Geometry check sheet. Reference: the model listing, model coordinates, mm. A direction names the side the tool comes from. Round coordinates to 2 decimals unless told otherwise and drop trailing zeros. Order: outer loops, then holes, each group sorted by start corner. A loop starts at its lowest first (then second) coordinate and runs counter-clockwise, first axis right, second up. Notation, with made-up numbers: M 5,29 L 41,29 A26 cw 41,45 Z; hole C 61,-9 d4. An arc over 180 degrees is marked long. Return JSON: item names as keys, results as strings. Group by question number.
```python
from build123d import *

# Parameters (mm, degrees)
F0_R            = 10
F0_R_2          = 8
F1_DEPTH        = 4
F3_DEPTH        = 3
F3_COPIES_COUNT = 3
F5_DEPTH        = 3
F5_COPIES_COUNT = 3
F7_DEPTH        = 3
F7_COPIES_COUNT = 3
F9_DEPTH        = 3
F9_COPIES_COUNT = 3
F10_W           = 0.5
F10_H           = 2
F10_W_2         = 3
F10_H_2         = 6


# Not quite as in the source:
# - a pattern or mirror of a feature is missing from the dataset's text; its kind, count and spacing are read off the source's solid


with BuildPart() as f1:
    # F0 (on Front) → F1 (new body, symmetric)
    with BuildSketch(Plane.XZ):
        Circle(F0_R)
        Circle(F0_R_2, mode=Mode.SUBTRACT)
    extrude(amount=F1_DEPTH, both=True)

    # F2 (on face) → F3 (cut)
    with BuildSketch(Plane.XZ.offset(4)):
        with BuildLine():
            Line((-0.525, 8.9827548503), (-0.525, 7.9827548503))
            ThreePointArc((-0.525, 7.9827548503), (0, 8), (0.525, 7.9827548503))
            Line((0.525, 7.9827548503), (0.525, 8.9827548503))
            Line((0.525, 8.9827548503), (-0.525, 8.9827548503))
        make_face()
    f3 = extrude(amount=-F3_DEPTH, mode=Mode.SUBTRACT)

    # F3_copies: F3 ×3 about axis
    f3_copies_axis = Axis((0, 0, 0), (0, 1, 0))
    for i in range(1, F3_COPIES_COUNT):
        add(f3.rotate(f3_copies_axis, i * 360 / F3_COPIES_COUNT), mode=Mode.SUBTRACT)

    # F4 (on Front) → F5 (cut)
    with BuildSketch(Plane.XZ):
        with BuildLine():
            ThreePointArc((6.6507684925, 4.4460407621), (6.9282032303, 4), (7.1757684925, 3.5367140882))
            Line((7.1757684925, 3.5367140882), (8.0417938963, 4.0367140882))
            Line((8.0417938963, 4.0367140882), (7.5167938963, 4.9460407621))
            Line((7.5167938963, 4.9460407621), (6.6507684925, 4.4460407621))
        make_face()
    f5 = extrude(amount=F5_DEPTH, mode=Mode.SUBTRACT)

    # F5_copies: F5 ×3 about axis
    f5_copies_axis = Axis((0, 0, 0), (0, 1, 0))
    for i in range(1, F5_COPIES_COUNT):
        add(f5.rotate(f5_copies_axis, i * 360 / F5_COPIES_COUNT), mode=Mode.SUBTRACT)

    # F6 (on face) → F7 (cut)
    with BuildSketch(Plane(origin=(0, 4, 0), x_dir=(-1, 0, 0), z_dir=(0, 1, 0))):
        with BuildLine():
            ThreePointArc((3.5367140882, 7.1757684925), (4, 6.9282032303), (4.4460407621, 6.6507684925))
            Line((4.4460407621, 6.6507684925), (4.9460407621, 7.5167938963))
            Line((4.9460407621, 7.5167938963), (4.0367140882, 8.0417938963))
            Line((4.0367140882, 8.0417938963), (3.5367140882, 7.1757684925))
        make_face()
    f7 = extrude(amount=-F7_DEPTH, mode=Mode.SUBTRACT)

    # F7_copies: F7 ×3 about axis
    f7_copies_axis = Axis((0, 0, 0), (0, 1, 0))
    for i in range(1, F7_COPIES_COUNT):
        add(f7.rotate(f7_copies_axis, i * 360 / F7_COPIES_COUNT), mode=Mode.SUBTRACT)

    # F8 (on Front) → F9 (cut)
    with BuildSketch(Plane.XZ):
        with BuildLine():
            ThreePointArc((-7.9827548503, -0.525), (-8, 0), (-7.9827548503, 0.525))
            Line((-7.9827548503, 0.525), (-8.9827548503, 0.525))
            Line((-8.9827548503, 0.525), (-8.9827548503, -0.525))
            Line((-8.9827548503, -0.525), (-7.9827548503, -0.525))
        make_face()
    f9 = extrude(amount=-F9_DEPTH, mode=Mode.SUBTRACT)

    # F9_copies: F9 ×3 about axis
    f9_copies_axis = Axis((0, 0, 0), (0, 1, 0))
    for i in range(1, F9_COPIES_COUNT):
        add(f9.rotate(f9_copies_axis, i * 360 / F9_COPIES_COUNT), mode=Mode.SUBTRACT)

    # F10 (on Right) → F11 (revolve)
    with BuildSketch(Plane.YZ):
        Polygon((4, 14), (4, 8), (5.75, 8), (5.75, 6.5), (11.5, 6.5), (11.5, 8), (8.3, 8), (8.3, 14), align=None)
        with Locations((0, 11)):
            Rectangle(F10_W, F10_H)
        with Locations((-5.5, 11)):
            Rectangle(F10_W_2, F10_H_2)
    revolve(axis=Axis((0, 0, 0), (0, -1, 0)))


solid = f1.part
```
Q1. Depth check by flat-ended pin: pin 1 Ø0.5 at (x, y) = (-8.5, 2) entering from -Z; pin 2 Ø0.7 at (x, z) = (-4.5, -7.5) entering from +Y; pin 3 Ø8 at (x, y) = (-5.5, 8) entering from -Z; pin 4 Ø4 at (x, z) = (3.5, 0) entering from -Y. Enter the tip coordinate at first touch or a pass-through.
Q2. Set-up check for faces 3 (the face through (8.5, 2.5, 0.525)), 4 (the face through (3.955, 8.665, -5.158)): record each of +Z, -Z, +X, -X, +Y, -Y from which the full face is reachable in a straight line by a thin tool's end or side.
Q3. Section check A-A on x = -10.75. Record the cut outline in (y, z).
Q4. Release check for a two-part mould opening along Z. For faces 1 (the face through (0.525, -1.5, -8.5)), 2 (the face through (9.54, 2.1, 3)) record: +Z half, -Z half, draft (parallel to the pull), parting line (faces both ways), or undercut.
Q5. Section check B-B on y = 2. Record the cut outline in (x, z) (3 decimals), plus the area to 3 significant figures.
Q6. Material ranges on line 1 along Y through (x, z) = (-8.75, 6.75); line 2 along X through (y, z) = (7, 0.25), recorded low to high.
Q7. Section check C-C on z = 11.25. Record the cut outline in (x, y), plus the area to 3 significant figures.
Geometry check:
{
 "1": {"pin 1": "stops at z = -5.65", "pin 2": "stops at y = 8.3", "pin 3": "stops at z = -13.92", "pin 4": "passes through"},
 "2": {"face 3": "none", "face 4": "+Y, -Y"},
 "3": {"outline": "M -7,-8.97 L -4,-8.97 L -4,8.97 L -7,8.97 Z; M -0.25,-5.33 L 0.25,-5.33 L 0.25,5.33 L -0.25,5.33 Z; M 4,-8.97 L 8.3,-8.97 L 8.3,8.97 L 4,8.97 Z"},
 "4": {"face 1": "undercut", "face 2": "parting line"},
 "5": {"outline": "C 0,0 d20; hole M -8.983,-0.525 L -7.983,-0.525 A8 ccw -4.446,-6.651 L -4.946,-7.517 L -4.037,-8.042 L -3.537,-7.176 A8 ccw 3.537,-7.176 L 4.037,-8.042 L 4.946,-7.517 L 4.446,-6.651 A8 ccw 7.983,-0.525 L 8.983,-0.525 L 8.983,0.525 L 7.983,0.525 A8 ccw 4.446,6.651 L 4.946,7.517 L 4.037,8.042 L 3.537,7.176 A8 ccw -3.537,7.176 L -4.037,8.042 L -4.946,7.517 L -4.446,6.651 A8 ccw -7.983,0.525 L -8.983,0.525 Z", "area": "107 mm^2"},
 "6": {"line 1": "y = -7 to -4, -0.25 to 0.25, 4 to 8.3", "line 2": "x = -14 to -6.5, 6.5 to 14"},
 "7": {"outline": "M -8.33,-7 L 8.33,-7 L 8.33,-4 L -8.33,-4 Z; M -8.33,4 L 8.33,4 L 8.33,8.3 L -8.33,8.3 Z; M -4.18,-0.25 L 4.18,-0.25 L 4.18,0.25 L -4.18,0.25 Z", "area": "126 mm^2"}
}
